Autodesk Inventor part; units mm, degrees
ref_plane "YZ Plane" through (0, 0, 0) normal (1, 0, 0) x (0, 1, 0)
ref_plane "XZ Plane" through (0, 0, 0) normal (0, 1, 0) x (-1, 0, 0)
ref_plane "XY Plane" through (0, 0, 0) normal (0, 0, 1) x (1, 0, 0)
sketch "Sketch1" plane through (0, 0, 0) normal (0, 1, 0) x (-1, 0, 0)
  line L0 (1, 0) -> (-6, 0)
  line L1 (0, -76.3) -> (0, 76.3)
  line L2 (0, -54.5) -> (-4, -54.5)
  line L3 (-4, -54.5) -> (-4, -36.5)
  line L4 (-4, -36.5) -> (-5, -36.5)
  line L5 (-5, -36.5) -> (-5, 36.5)
  line L6 (-5, 36.5) -> (-4, 36.5)
  line L7 (-4, 36.5) -> (-4, 54.5)
  line L8 (-4, 54.5) -> (0, 54.5)
  dimension "d1" = 18
  dimension "d2" = 8
  dimension "d3" = 10
  dimension "d5" = 8
  dimension "d8" = 18
  dimension "d9" = 73
revolve "Revolution1" add sketch "Sketch1" angle 360 about axis through (0, 0, -10) along (0, 0, 1)
chamfer "Chamfer1" distance 0.5 angle 45 4 edges at (-4, 0, -54.5) (-4, 0, 54.5) (-5, 0, 36.5) (-5, 0, -36.5)
thread "Thread1"
thread "Thread2"
equation "\"d5\" = d2"
equation "\"d8\" = d1"
properties part number "Rear Wheel Axle"
Could you check a few things on this model? Use its own coordinates, in mm. A direction names the side the tool comes from. Round coordinates to 2 decimals unless told otherwise and drop trailing zeros. Write each loop counter-clockwise with the first axis right and the second up, starting at its lowest first coordinate (ties: lowest second). Pieces come first, ordered by that corner, then holes. Notation, with made-up numbers: M 47,77 L 77,77 A10 ccw 77,89 Z; hole C 46,-14 d7. An arc over 180 degrees is marked long. Answer in a Markdown table with one row per item. Add a question column.
Q1. Imagine slicing it at A-A (x = 0). Please give me the cut outline in (y, z), then the cut area to 3 significant figures.
Q2. On a 3-axis mill with a long thin cutter (end or side, diameter ignored), from which of +Z, -Z, +X, -X, +Y, -Y can I reach the whole of each face in a straight line? I mean faces 1 (the cylindrical face through (-1.08, -4.88, 0.5)), 2 (the flat face through (-3, -3, 36.5)), 3 (the flat face through (-3, -3, -36.5)). Say none if no direction works.
Q3. Will these pins go through, and if not, where does the flat tip stop? pin 1 Ø2 at (x, z) = (1, 9.5) entering from -Y; pin 2 Ø4 at (x, z) = (4, 41.5) entering from +Y; pin 3 Ø5 at (y, z) = (2.5, -38) entering from -X; pin 4 Ø1.5 at (x, z) = (-3.5, 13.5) entering from +Y.
Q4. If I drill on line 1 (Y direction, x = -0.25, z = -11); line 2 (Y direction, x = 3, z = -32), over which ranges is the centre line in solid material (lowest first)? Write a range as from..to.
Q5. Imagine slicing it at B-B (z = -28). Please give me the cut outline in (x, y), then the cut area to 3 significant figures.
Values:
| question | item | result |
|---|---|---|
| 1 | outline | M -5,-36 L -4.5,-36.5 L -4,-36.5 L -4,-54 L -3.5,-54.5 L 3.5,-54.5 L 4,-54 L 4,-36.5 L 4.5,-36.5 L 5,-36 L 5,36 L 4.5,36.5 L 4,36.5 L 4,54 L 3.5,54.5 L -3.5,54.5 L -4,54 L -4,36.5 L -4.5,36.5 L -5,36 Z |
| 1 | area | 1,020 mm^2 |
| 2 | face 1 | +Z, -Z |
| 2 | face 2 | +Z |
| 2 | face 3 | -Z |
| 3 | pin 1 | y = -5 |
| 3 | pin 2 | y = 3.46 |
| 3 | pin 3 | x = -4.9 |
| 3 | pin 4 | y = 4.18 |
| 4 | line 1 | -4.99..4.99 |
| 4 | line 2 | -4..4 |
| 5 | outline | C 0,0 d10 |
| 5 | area | 78.5 mm^2 |
